from build123d import *

# Parameters (mm, degrees)
SKETCH_1_R                           = 5
SKETCH_1_R_2                         = 3
HUB_OD10_ID6_L10_DEPTH               = 10
SKETCH_2_R                           = 11
SKETCH_2_R_2                         = 3
FLANGE_OD22_T2P2_DEPTH               = 2.2
SKETCH_3_R                           = 1.5
F_4XD3_ON_PCD16_DEPTH                = 2.2
SKETCH_4_R                           = 1.25
M3_GRUB_SCREW_RADIAL_REFERENCE_DEPTH = 2.1


with BuildPart() as part:
    # 草图1 → Hub_OD10_ID6_L10 (new body)
    with BuildSketch(Plane.XY):
        Circle(SKETCH_1_R)
        Circle(SKETCH_1_R_2, mode=Mode.SUBTRACT)
    extrude(amount=HUB_OD10_ID6_L10_DEPTH)

    # 草图2 → Flange_OD22_T2p2 (add)
    with BuildSketch(Plane.XY.offset(10)):
        Circle(SKETCH_2_R)
        Circle(SKETCH_2_R_2, mode=Mode.SUBTRACT)
    extrude(amount=FLANGE_OD22_T2P2_DEPTH)

    # 草图3 → 4xD3_on_PCD16 (cut)
    with BuildSketch(Plane.XY.offset(12.2)):
        with Locations((8, 0)):
            Circle(SKETCH_3_R)
        with Locations((0, 8)):
            Circle(SKETCH_3_R)
        with Locations((-8, 0)):
            Circle(SKETCH_3_R)
        with Locations((0, -8)):
            Circle(SKETCH_3_R)
    extrude(amount=-F_4XD3_ON_PCD16_DEPTH, mode=Mode.SUBTRACT)

    # 草图4 → M3_grub_screw_radial_reference (cut)
    with BuildSketch(Plane(origin=(5, 0, 0), x_dir=(0, 0, -1), z_dir=(1, 0, 0))):
        with Locations((-5, 0)):
            Circle(SKETCH_4_R)
    extrude(amount=-M3_GRUB_SCREW_RADIAL_REFERENCE_DEPTH, mode=Mode.SUBTRACT)


solid = part.part
Build history of the part. All positions in model axes, mm. A direction names the side the tool comes from. Round coordinates to 2 decimals unless told otherwise and drop trailing zeros. Write each loop counter-clockwise with the first axis right and the second up, starting at its lowest first coordinate (ties: lowest second). Pieces come first, ordered by that corner, then holes. Notation, with made-up numbers: M 75.5,-30 L 125.5,-30 A24 cw 125.5,-6 Z; hole C 45,26 d11. An arc over 180 degrees is marked long. Answer in a Markdown table with one row per item.
1. Saw through at C-C (z = 9.25). List the corners of the cut face in (x, y).
Geometry check:
| item | result |
|---|---|
| outline | C 0,0 d10; hole C 0,0 d6 |
2. Saw through at D-D (y = 7.5). List the corners of the cut face in (x, z), and give its area (3 significant figures).
Geometry check:
| item | result |
|---|---|
| outline | M -8.05,10 L -1.41,10 L -1.41,12.2 L -8.05,12.2 Z; M 1.41,10 L 8.05,10 L 8.05,12.2 L 1.41,12.2 Z |
| area | 29.2 mm2 |
3. Flat gauge pins, fed straight in: P1, Ø1, axis at x = -4.5, z = 5, coming from the -Y side; P2, Ø2, axis at y = 0, z = 5, coming from the +X side; P3, Ø1.5, axis at x = -4.5, z = 4.5, coming from the +Y side. Where does each tip first touch, or does it go through?
Geometry check:
| item | result |
|---|---|
| P1 | y = -3 |
| P2 | x = 2.9 |
| P3 | y = 3.31 |
4. Saw through at B-B (y = 0). List the corners of the cut face in (x, z), and give its area (3 significant figures).
Geometry check:
| item | result |
|---|---|
| outline | M -11,10 L -9.5,10 L -9.5,12.2 L -11,12.2 Z; M -6.5,10 L -5,10 L -5,0 L -3,0 L -3,12.2 L -6.5,12.2 Z; M 3,0 L 5,0 L 5,3.75 L 3,3.75 Z; M 3,6.25 L 5,6.25 L 5,10 L 6.5,10 L 6.5,12.2 L 3,12.2 Z; M 9.5,10 L 11,10 L 11,12.2 L 9.5,12.2 Z |
| area | 57.0 mm2 |
5. Saw through at A-A (x = 0). List the corners of the cut face in (y, z).
Geometry check:
| item | result |
|---|---|
| outline | M -11,10 L -9.5,10 L -9.5,12.2 L -11,12.2 Z; M -6.5,10 L -5,10 L -5,0 L -3,0 L -3,12.2 L -6.5,12.2 Z; M 3,0 L 5,0 L 5,10 L 6.5,10 L 6.5,12.2 L 3,12.2 Z; M 9.5,10 L 11,10 L 11,12.2 L 9.5,12.2 Z |
6. Mould opens along X. For faces 4 (the face through (-9.5, 0.07, 11.12)), 5 (the face through (6.5, 0.07, 11.12)), 6 (the face through (-2.38, -10.74, 11.08)), 7 (the face through (2.3, -2.3, 12.2)) say: +X half, -X half, draft (parallel to the pull), parting line (faces both ways), or undercut.
Geometry check:
| item | result |
|---|---|
| face 4 | undercut |
| face 5 | undercut |
| face 6 | parting line |
| face 7 | draft |
7. Which spindle directions (+Z, -Z, +X, -X, +Y, -Y) get a long thin tool onto all of the face, cutting with end or side? Do faces 1 (the face through (3.96, 0.05, 6.25)), 2 (the face through (-0.325, 6.536, 11.115)), 3 (the face through (5, -2, 10)). Say none if no direction does.
Geometry check:
| item | result |
|---|---|
| face 1 | +X |
| face 2 | +Z, -Z |
| face 3 | -Z |
8. Probe L1, parallel to Y at x = 0, z = 11.7; L2, parallel to Y at x = 0, z = 6; L3, parallel to Z at x = 3.7, y = 0. List the from-to ranges inside material, lowest first. Write a range as [from, to].
Geometry check:
| item | result |
|---|---|
| L1 | [-11, -9.5], [-6.5, -3], [3, 6.5], [9.5, 11] |
| L2 | [-5, -3], [3, 5] |
| L3 | [0, 3.75], [6.25, 12.2] |
